```python
from build123d import *

# Parameters (mm, degrees)
SKETCH_1_R      = 5
EXTRUDE_1_DEPTH = 4


with BuildPart() as part:
    # 草图1 → 凸台-拉伸1 (new body)
    with BuildSketch(Plane.XY):
        with BuildLine():
            Line((428.542857143, -15.145714286), (348.542857143, -30.145714286))
            Line((348.542857143, -30.145714286), (-1.457142857, -30.145714286))
            ThreePointArc((-1.457142857, -30.145714286), (-31.457142857, -0.145714286), (-1.457142857, 29.854285714))
            Line((-1.457142857, 29.854285714), (348.542857143, 29.854285714))
            Line((348.542857143, 29.854285714), (428.542857143, 14.854285714))
            ThreePointArc((428.542857143, 14.854285714), (443.542857143, -0.145714286), (428.542857143, -15.145714286))
        make_face()
        with Locations((428.542857143, -0.145714286)):
            Circle(SKETCH_1_R, mode=Mode.SUBTRACT)
        with Locations((-1.457142857, -0.145714286)):
            Circle(SKETCH_1_R, mode=Mode.SUBTRACT)
        with Locations((348.542857143, -0.145714286)):
            Circle(SKETCH_1_R, mode=Mode.SUBTRACT)
    extrude(amount=EXTRUDE_1_DEPTH)


solid = part.part
```
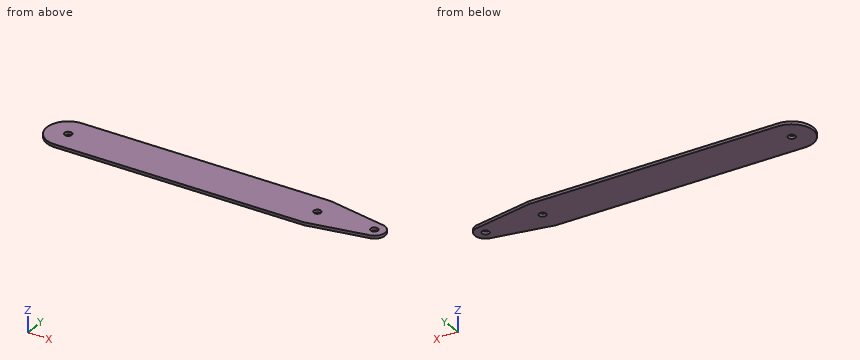
Design review of the part built by this model. Coordinates are the model's own, in mm. Give positions to 0.01 mm unless a question says otherwise; leave off trailing zeros. Order: outer loops, then holes, each group sorted by start corner. A loop starts at its lowest first (then second) coordinate and runs counter-clockwise, first axis right, second up. Notation, with made-up numbers: (64.25, 59.25) -> (116.25, 59.25) arc R30 cw to (116.25, 92.25) -> close; hole circle Ø1 at (51, 53.5). An arc over 180 degrees is marked (long way). Write each question's results on one line, items separated by ' | '. Start each with the question number.
Q1. Add section C-C on y = 22.5. Give the boundary of the cut face in (x, z).
Q2. Add section A-A on z = 1.4. Give the boundary of the cut face in (x, y), and give its area (3 significant figures).
Q3. Wall thickness on L1, parallel to X at y = 4, z = 1.3; L2, parallel to Y at x = 390.5, z = 2.9; L3, parallel to X at y = -9, z = 0.5: over which ranges is each line inside the solid? List them lowest first. Write a range as from..to.
Q4. For pin 1 (1.5 mm diameter, centred on x = 378.5, z = 3, fed in from +Y), flat-tipped, find the tip position at first contact; note if it passes through.
Q5. Add section B-B on y = -20. Give the boundary of the cut face in (x, z).
Found:
1) outline: (-21.13, 0) -> (387.77, 0) -> (387.77, 4) -> (-21.13, 4) -> close
2) outline: (-1.46, -30.15) -> (348.54, -30.15) -> (428.54, -15.15) arc R15 ccw to (428.54, 14.85) -> (348.54, 29.85) -> (-1.46, 29.85) arc R30 ccw to start; hole circle Ø10 at (-1.46, -0.15); hole circle Ø10 at (348.54, -0.15); hole circle Ø10 at (428.54, -0.15) | area: 26,100 mm2
3) L1: x = -31.17..-4.25, 1.34..345.75, 351.34..425.75, 431.34..442.96 | L2: y = -22.28..21.99 | L3: x = -30.12..440.65
4) pin 1: stops at y = 24.38
5) outline: (-23.95, 0) -> (402.65, 0) -> (402.65, 4) -> (-23.95, 4) -> close
